Geometry: see drawing. Coordinates: mm, zero at the bounding-box minimum. Give positions to 0.01 mm unless a question says otherwise; leave off trailing zeros. Write each loop counter-clockwise with the first axis right and the second up, starting at its lowest first coordinate (ties: lowest second). Pieces come first, ordered by that corner, then holes. Notation, with made-up numbers: (80.25, -10) -> (94.25, -10) arc R36 cw to (94.25, 29) -> close; hole circle Ø6 at (-38.75, -25). An arc over 180 degrees is marked (long way). Use one line per item in the form item = value. Start each with the question number.
(1) Cut plane B-B, the plane z = 38.1. Output: boundary loops of the cut face in (x, y) (3 decimals), and give its area (3 significant figures).
(2) Material intervals for line 1 along X through (y, z) = (0.75, 38.1) (3 decimals); line 2 along X through (y, z) = (0.4, 36.5), sorted ascending. Write a range as from..to.
(3) Cut plane A-A, the plane x = 38.1. Output: boundary loops of the cut face in (y, z) (3 decimals), and give its area (3 significant figures).
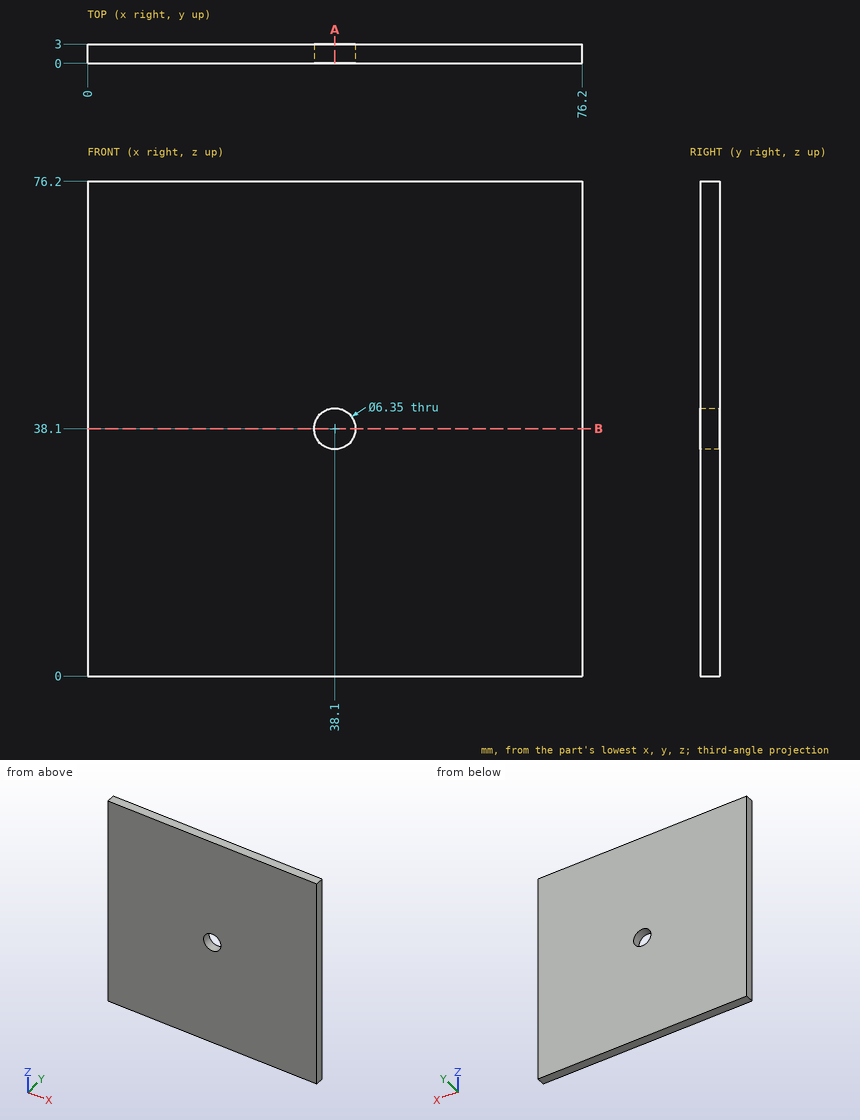
Geometry says:
q1.outline = (0, 0) -> (34.925, 0) -> (34.925, 3) -> (0, 3) -> close; (41.275, 0) -> (76.2, 0) -> (76.2, 3) -> (41.275, 3) -> close
q1.area = 210 mm^2
q2.line_1 = 0..34.925, 41.275..76.2
q2.line_2 = 0..35.36, 40.84..76.2
q3.outline = (0, 0) -> (3, 0) -> (3, 34.925) -> (0, 34.925) -> close; (0, 41.275) -> (3, 41.275) -> (3, 76.2) -> (0, 76.2) -> close
q3.area = 210 mm^2
